```python
from build123d import *

# Parameters (mm, degrees)
F1_DEPTH  = 1.6002
F4_DEPTH  = 2.159
F6_DEPTH  = 13.081
F7_R      = 2.5019
F8_DEPTH  = 16.8412
F9_R      = 0.8001
F9_R_2    = 0.79375
F10_DEPTH = 16.8412


with BuildPart() as f1:
    # F0 (on Top) → F1 (new body)
    with BuildSketch(Plane.XY):
        with BuildLine():
            Line((1.433722, 7.6962), (-1.433722, 7.6962))
            Line((-1.433722, 7.6962), (-25.9207, 7.6962))
            ThreePointArc((-25.9207, 7.6962), (-33.6169, 0), (-25.9207, -7.6962))
            Line((-25.9207, -7.6962), (-1.433722, -7.6962))
            Line((-1.433722, -7.6962), (1.433722, -7.6962))
            Line((1.433722, -7.6962), (25.9207, -7.6962))
            ThreePointArc((25.9207, -7.6962), (33.6169, 0), (25.9207, 7.6962))
            Line((25.9207, 7.6962), (1.433722, 7.6962))
        make_face()
    extrude(amount=F1_DEPTH)



with BuildPart() as f4:
    # F3 (on offset) → F4 (new body)
    with BuildSketch(Plane.XY.offset(-13.081)):
        with BuildLine():
            Line((-35.865766, -7.429749), (-6.35, -15.4051))
            Line((-6.35, -15.4051), (6.35, -15.4051))
            Line((6.35, -15.4051), (35.865766, -7.429749))
            ThreePointArc((35.865766, -7.429749), (41.487496, 1.012586), (33.8582, 7.6962))
            Line((33.8582, 7.6962), (0, 7.6962))
            Line((0, 7.6962), (-33.8582, 7.6962))
            ThreePointArc((-33.8582, 7.6962), (-41.487496, 1.012586), (-35.865766, -7.429749))
        make_face()
    extrude(amount=-F4_DEPTH)


with BuildPart() as f1_1:
    add(f1.part)

    add(f4.part)  # F6 merges F4
    # F5 (on face) → F6 (join, through all)
    with BuildSketch(Plane(origin=(0, 0, 0), x_dir=(1, 0, 0), z_dir=(0, 0, -1))):
        with BuildLine():
            Line((0, -3.1369), (26.7081, -3.1369))
            ThreePointArc((26.7081, -3.1369), (29.845, 0), (26.7081, 3.1369))
            Line((26.7081, 3.1369), (0, 3.1369))
            Line((0, 3.1369), (-26.7081, 3.1369))
            ThreePointArc((-26.7081, 3.1369), (-29.845, 0), (-26.7081, -3.1369))
            Line((-26.7081, -3.1369), (0, -3.1369))
        make_face()
    extrude(amount=F6_DEPTH)

    # F7 (on face) → F8 (cut, through all)
    with BuildSketch(Plane.XY.offset(1.6002)):
        with Locations((-5.23875, 0)):
            Circle(F7_R)
        with Locations((-15.71625, 0)):
            Circle(F7_R)
        with Locations((-26.19375, 0)):
            Circle(F7_R)
        with Locations((5.23875, 0)):
            Circle(F7_R)
        with Locations((15.71625, 0)):
            Circle(F7_R)
        with Locations((26.19375, 0)):
            Circle(F7_R)
    extrude(amount=-F8_DEPTH, mode=Mode.SUBTRACT)

    # F9 (on face) → F10 (cut, through all)
    with BuildSketch(Plane(origin=(0, 0, -15.24), x_dir=(1, 0, 0), z_dir=(0, 0, -1))):
        with Locations((38.354, 0)):
            Circle(F9_R)
        with Locations((-38.354, 0)):
            Circle(F9_R)
        with Locations((-6.35, 12.309221)):
            Circle(F9_R_2)
        with Locations((0, 10.297953)):
            Circle(F9_R_2)
        with Locations((6.35, 12.309221)):
            Circle(F9_R_2)
    extrude(amount=-F10_DEPTH, mode=Mode.SUBTRACT)


solid = f1_1.part
```
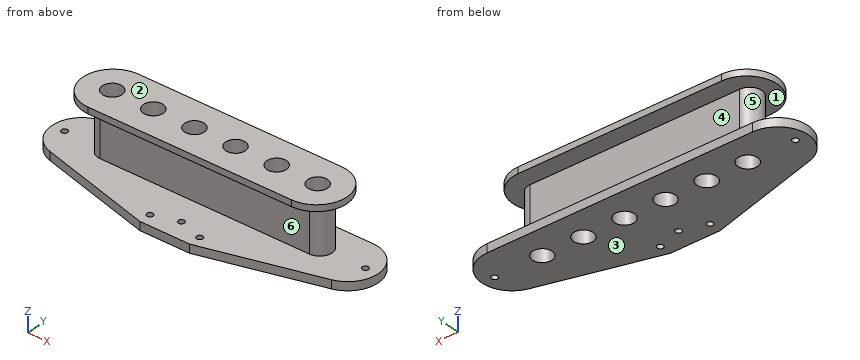
CAD build for the part. Positions are in the model's coordinates, mm. Face numbers are marked on the shaded views. A direction names the side the tool comes from. Round coordinates to 2 decimals unless told otherwise and drop trailing zeros. Write each loop counter-clockwise with the first axis right and the second up, starting at its lowest first coordinate (ties: lowest second). Pieces come first, ordered by that corner, then holes.
Item 1: Drill centre lines: L1, parallel to Y at x = 6.35, z = -14.1; L2, parallel to Z at x = -22.5, y = -6.25; L3, parallel to Z at x = -15, y = -8. Where is each one in solid material? Low to high.
Filled in:
L1: y = -15.41 to -13.1, -11.52 to -2.24, 2.24 to 7.7
L2: z = -15.24 to -13.08, 0 to 1.6
L3: z = -15.24 to -13.08
Item 2: Band-saw the part on B-B on y = 0. Give the number of separate pieces and of enclosed holes in the cut face, then the cut area to 3 significant figures.
Filled in:
separate pieces: 9
enclosed holes: 0
area: 555 mm2
Item 3: Mould opens along Z. For the marked faces 1, 2 and 3 say: released by +Z, released by -Z, zero draft, split by the parting line, or undercut.
Filled in:
face 1: undercut
face 2: released by +Z
face 3: released by -Z
Item 4: Drop flat-ended pins along their axis: pin 1 Ø1.3 at (x, y) = (0, -10.3) entering from -Z (3 decimals); pin 2 Ø10 at (x, z) = (31, -6) entering from -Y; pin 3 Ø6 at (x, y) = (-5.24, 0) entering from -Z; pin 4 Ø3 at (x, z) = (26.5, -9.5) entering from +Y. Give the stop position or say it passes through.
Filled in:
pin 1: passes through
pin 2: stops at y = -3.14
pin 3: stops at z = -15.24
pin 4: stops at y = 3.14
Item 5: Band-saw the part on A-A on z = -7. Write the cut outline in (x, y), then the cut area to 3 significant figures.
Filled in:
outline: (-26.71, -3.14) - (26.71, -3.14) arc R3.14 ccw to (26.71, 3.14) - (-26.71, 3.14) arc R3.14 ccw to start; hole circle Ø5 at (-26.19, 0); hole circle Ø5 at (-15.72, 0); hole circle Ø5 at (-5.24, 0); hole circle Ø5 at (5.24, 0); hole circle Ø5 at (15.72, 0); hole circle Ø5 at (26.19, 0)
area: 248 mm2
Item 6: Band-saw the part on C-C on x = 15. Write the cut outline in (y, z).
Filled in:
outline: (-13.07, -15.24) - (-2.4, -15.24) - (-2.4, 1.6) - (-7.7, 1.6) - (-7.7, 0) - (-3.14, 0) - (-3.14, -13.08) - (-13.07, -13.08) - close; (2.4, -15.24) - (7.7, -15.24) - (7.7, -13.08) - (3.14, -13.08) - (3.14, 0) - (7.7, 0) - (7.7, 1.6) - (2.4, 1.6) - close
Item 7: Tool access for the marked faces 4, 5 and 6: list every direction of +Z, -Z, +X, -X, +Y, -Y with a clear straight run to the whole face (end or side of a thin tool).
Filled in:
face 4: +X, -X, +Y
face 5: -X
face 6: +X, -X, -Y
Item 8: Band-saw the part on D-D on x = -27.5. Write the cut outline in (y, z), then the cut area to 3 significant figures.
Filled in:
outline: (-9.69, -15.24) - (-2.13, -15.24) - (-2.13, 1.6) - (-7.53, 1.6) - (-7.53, 0) - (-3.04, 0) - (-3.04, -13.08) - (-9.69, -13.08) - close; (2.13, -15.24) - (7.7, -15.24) - (7.7, -13.08) - (3.04, -13.08) - (3.04, 0) - (7.53, 0) - (7.53, 1.6) - (2.13, 1.6) - close
area: 69.2 mm2
